The listing builds one solid part. Answer for the finished solid, in the listing's coordinates (mm). A direction names the side the tool comes from. Give positions to 0.01 mm unless a question says otherwise; leave off trailing zeros. Loops run counter-clockwise (first coordinate to the right, second up) from the corner with the lowest first, then second, coordinate; pieces in that order, holes last. Notation, with made-up numbers: (37.5, -18.5) -> (42.5, -18.5) arc R11 cw to (42.5, -13.5) -> close; hole circle Ø1 at (37, 30). An arc over 180 degrees is marked (long way). One line per question, with ' | ' between items. Start each with the question number.
from build123d import *

# Parameters (mm, degrees)
F0_R     = 26.2781927152
F1_DEPTH = 12.7
F3_W     = 72.8053152561
F3_H     = 72.0469206572
F4_DEPTH = 5.08


# Not quite as in the source:
# - a fillet or chamfer that OpenCascade refuses, or shapes differently, is made with other operations: its cross-section is extruded or revolved along the edge and cut away or added


with BuildPart() as f1:
    # F0 (on Top) → F1 (new body)
    with BuildSketch(Plane.XY):
        Circle(F0_R)
    extrude(amount=F1_DEPTH)

    # F2: fillet of radius 25.4 on 1 edges, made by hand

    # F2_s1 → F2_t2 (revolve, cut)
    with BuildSketch(Plane.XZ):
        with BuildLine():
            ThreePointArc((26.2781927152, 0), (16.9811474591, 9.2970452561), (4.2811474591, 12.7))
            Line((4.2811474591, 12.7), (26.2781927152, 12.7))
            Line((26.2781927152, 12.7), (26.2781927152, 0))
        make_face()
    revolve(axis=Axis((0, 0, 12.7), (0, 0, 1)), mode=Mode.SUBTRACT)

    # F3 (on Top) → F4 (join)
    with BuildSketch(Plane.XY):
        Rectangle(F3_W, F3_H)
    extrude(amount=-F4_DEPTH)


solid = f1.part
1. Each of these flat-tipped pins is pushed along its axis until it touches: pin 1 Ø1 at (y, z) = (5.5, 7.5) entering from -X; pin 2 Ø1 at (y, z) = (7.5, 3) entering from +X; pin 3 Ø8 at (y, z) = (5.5, 8.5) entering from +X. Where does it stop, or does it pass through?
2. The part is cut by section A-A (x = -30). Write down the section's boundary in (y, z), plus the area to 3 significant figures.
3. For faces 1 (the flat face through (-36.403, -1, -3)), 2 (the flat face through (16, 25, 0)), determine the directions among +Z, -Z, +X, -X, +Y, -Y from which every point of the face is accessible in a straight line to the end or side of a thin tool.
4. Straight lines are drawn through the part: L1, parallel to Z at x = -28.5, y = 1; L2, parallel to Z at x = -21.5, y = 7; L3, parallel to X at y = -14, z = 5.75. For each, find the intervals that lie inside material, in ascending order.
5. The part is cut by section B-B (y = 31.5). Write down the section's boundary in (x, z).
Check sheet entries:
1) pin 1: stops at x = -19.57 | pin 2: stops at x = 23.49 | pin 3: stops at x = 22.41
2) outline: (-36.02, -5.08) -> (36.02, -5.08) -> (36.02, 0) -> (-36.02, 0) -> close | area: 366 mm^2
3) face 1: +Z, -Z, -X, +Y, -Y | face 2: +Z
4) L1: z = -5.08 to 0 | L2: z = -5.08 to 4.88 | L3: x = -16.63 to 16.63
5) outline: (-36.4, -5.08) -> (36.4, -5.08) -> (36.4, 0) -> (-36.4, 0) -> close
